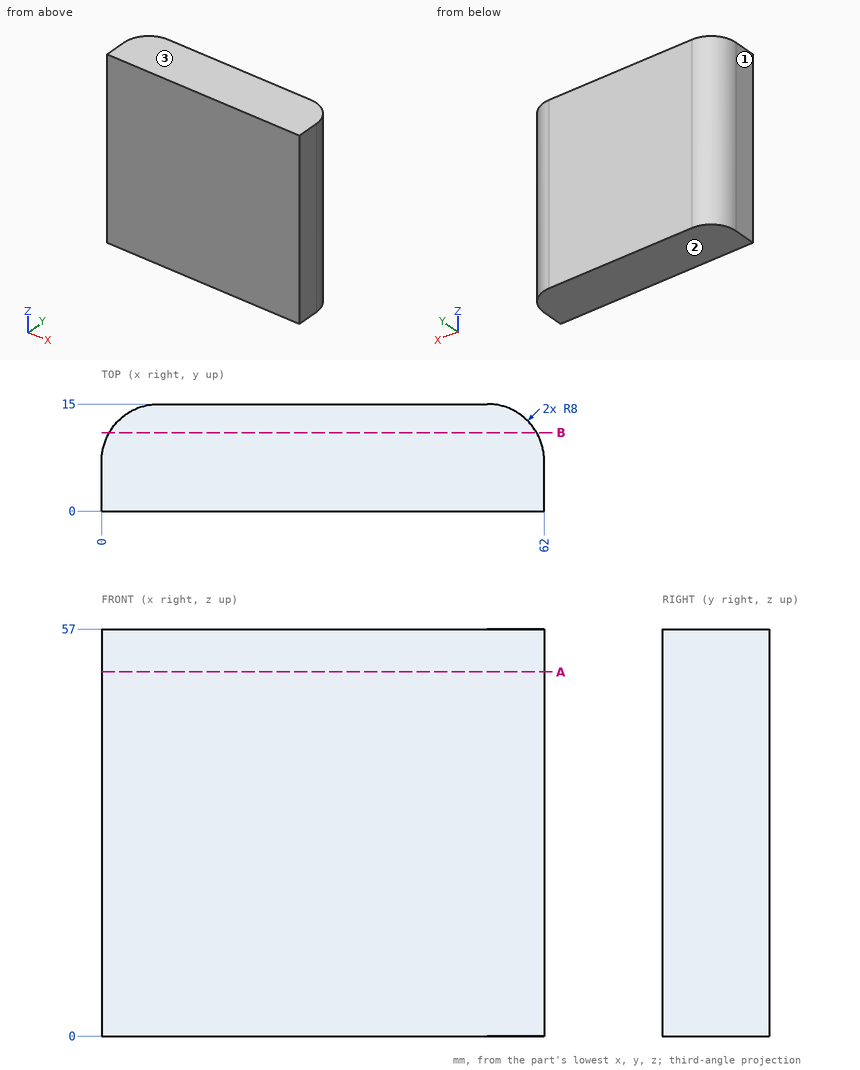
Geometry check sheet. Reference: drawing and pictorial views, mm from the part's lowest x, y, z. Give positions to 0.01 mm unless a question says otherwise; leave off trailing zeros. Write each loop counter-clockwise with the first axis right and the second up, starting at its lowest first coordinate (ties: lowest second). Pieces come first, ordered by that corner, then holes. Notation, with made-up numbers: (25.25, 63) -> (78.25, 63) arc R32 ccw to (78.25, 89) -> close; hole circle Ø3 at (76.25, 57). An arc over 180 degrees is marked (long way). One line per item, written item: value. Start each with the question number.
Item 1: Section check B-B on y = 11. Record the cut outline in (x, z).
Item 2: Section check A-A on z = 51. Record the cut outline in (x, y), then the cut area to 3 significant figures.
Item 3: Gauge pin test, flat ends, axial feed: pin 1 (1.5 mm diameter, centred on x = 16.5, y = 10, fed in from -Z); pin 2 (1.5 mm diameter, centred on y = 13, z = 13, fed in from -X). Record the tip position at first contact, or that the pin passes through.
Item 4: Material ranges on probe 1 along X at (y, z) = (10.5, 44); probe 2 along X at (y, z) = (9.25, 27.5); probe 3 along Y at (x, z) = (56, 38.5), recorded low to high. Write a range as from..to.
Item 5: Draft check along Z on the marked faces 1, 2 and 3. Enter one of: +Z half, -Z half, draft (parallel to the pull), parting line (faces both ways), or undercut.
Results list:
1. outline: (1.07, 0) -> (60.93, 0) -> (60.93, 57) -> (1.07, 57) -> close
2. outline: (0, 0) -> (62, 0) -> (62, 7) arc R8 ccw to (54, 15) -> (8, 15) arc R8 ccw to (0, 7) -> close
2. area: 903 mm²
3. pin 1: z = 0
3. pin 2: x = 1.96
4. probe 1: 0.81..61.19
4. probe 2: 0.32..61.68
4. probe 3: 0..14.75
5. face 1: draft
5. face 2: -Z half
5. face 3: +Z half
